CAD build for the part. Positions are in the model's coordinates, mm. Face numbers are marked on the shaded views. A direction names the side the tool comes from. Give positions to 0.01 mm unless a question says otherwise; leave off trailing zeros. Loops run counter-clockwise (first coordinate to the right, second up) from the corner with the lowest first, then second, coordinate; pieces in that order, holes last. Notation, with made-up numbers: (-1, -29) - (26, -29) arc R13 ccw to (26, -6) - close; hole circle Ø3 at (74, 59). An arc over 180 degrees is marked (long way). Return JSON: item names as keys, results as strings.
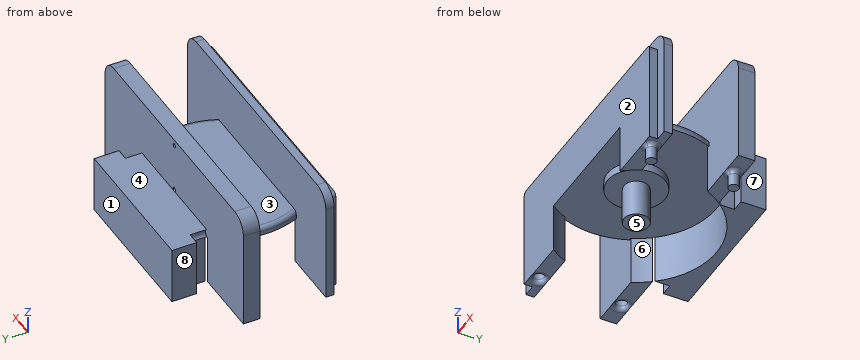
from build123d import *

# Parameters (mm, degrees)
BOSS_EXTRUDE1_DEPTH     = 1
SKETCH2_R               = 1.51
BOSS_EXTRUDE2_DEPTH     = 5.5
SKETCH3_R               = 3.5
BOSS_EXTRUDE3_DEPTH     = 1
SKETCH4_W               = 2
SKETCH4_H               = 17
BOSS_EXTRUDE4_DEPTH     = 6
SKETCH5_W               = 18
SKETCH5_H               = 2
BOSS_EXTRUDE5_DEPTH     = 6
SKETCH6_W               = 7
SKETCH6_H               = 2
BOSS_EXTRUDE6_DEPTH     = 5
BOSS_EXTRUDE7_DEPTH     = 6
CUT_EXTRUDE1_DEPTH      = 21.639767441
SKETCH9_W               = 2.937742252
SKETCH9_H               = 8
CUT_EXTRUDE2_DEPTH      = 6
CUT_EXTRUDE11_START     = -6
SKETCH21_R              = 9.75
SKETCH21_R_2            = 3.5
CUT_EXTRUDE11_DEPTH     = 6
SKETCH10_W              = 32
SKETCH10_H              = 2
BOSS_EXTRUDE8_DEPTH     = 7
FILLET1_R               = 0.5
SKETCH11_R              = 0.625
BOSS_EXTRUDE9_DEPTH     = 2
SKETCH14_W              = 3.5
SKETCH14_H              = 2
CUT_EXTRUDE5_DEPTH      = 24.937418532
SKETCH12_R              = 0.675
CUT_EXTRUDE3_DEPTH      = 2.5
CUT_EXTRUDE6_DEPTH      = 2
FILLET2_R               = 0.5
FILLET3_R               = 0.5
FILLET4_R               = 2
CUT_EXTRUDE7_DEPTH      = 25.677925456
CUT_EXTRUDE7_DEPTH_BACK = 1
SKETCH19_R              = 0.25
CUT_EXTRUDE9_DEPTH      = 2
SKETCH20_W              = 2
SKETCH20_H              = 3
CUT_EXTRUDE10_DEPTH     = 24.937418532


with BuildPart() as part:
    # Sketch1 → Boss-Extrude1 (new body)
    with BuildSketch(Plane.XY):
        Polygon((-11, 6), (-11, 11), (11, 11), (11, 6), (11, -6), (-11, -6), align=None)
    extrude(amount=BOSS_EXTRUDE1_DEPTH)

    # Sketch2 → Boss-Extrude2 (add)
    with BuildSketch(Plane(origin=(0, 0, 0), x_dir=(-1, 0, 0), z_dir=(0, 0, -1))):
        with Locations(Location((0, 0, 0), (0, 0, 180))):
            Circle(SKETCH2_R)
    extrude(amount=BOSS_EXTRUDE2_DEPTH)

    # Sketch3 → Boss-Extrude3 (add)
    with BuildSketch(Plane(origin=(0, 0, 0), x_dir=(-1, 0, 0), z_dir=(0, 0, -1))):
        with Locations(Location((0, 0, 0), (0, 0, 180))):
            Circle(SKETCH3_R)
    extrude(amount=BOSS_EXTRUDE3_DEPTH)

    # Sketch4 → Boss-Extrude4 (add)
    with BuildSketch(Plane(origin=(0, 0, 0), x_dir=(-1, 0, 0), z_dir=(0, 0, -1))):
        with Locations((10, 2.5)):
            Rectangle(SKETCH4_W, SKETCH4_H)
        with Locations((-10, 2.5)):
            Rectangle(SKETCH4_W, SKETCH4_H)
    extrude(amount=BOSS_EXTRUDE4_DEPTH)

    # Sketch5 → Boss-Extrude5 (add)
    with BuildSketch(Plane(origin=(0, 0, 0), x_dir=(-1, 0, 0), z_dir=(0, 0, -1))):
        with Locations((0, 10)):
            Rectangle(SKETCH5_W, SKETCH5_H)
    extrude(amount=BOSS_EXTRUDE5_DEPTH)

    # Sketch6 → Boss-Extrude6 (add)
    with BuildSketch(Plane(origin=(11, 0, 0), x_dir=(0, 0, -1), z_dir=(1, 0, 0))):
        with Locations((2.5, -5)):
            Rectangle(SKETCH6_W, SKETCH6_H)
        with Locations((2.5, 5)):
            Rectangle(SKETCH6_W, SKETCH6_H)
    boss_extrude6 = extrude(amount=BOSS_EXTRUDE6_DEPTH)

    # Mirror1: Boss-Extrude6 across plane
    add(boss_extrude6.mirror(Plane(origin=(0, 0, 0), x_dir=(0, 0, 1), z_dir=(1, 0, 0))))

    # Sketch7 → Boss-Extrude7 (add)
    with BuildSketch(Plane(origin=(0, 0, -6), x_dir=(-1, 0, 0), z_dir=(0, 0, -1))):
        with BuildLine():
            ThreePointArc((-6.708203932, -6), (-8.407551231, -3.211398808), (-9, 0))
            Line((-9, 0), (-9, -6))
            Line((-9, -6), (-6.708203932, -6))
        make_face()
        with BuildLine():
            Line((-9, 9), (-9, 0))
            ThreePointArc((-9, 0), (-6.363961031, 6.363961031), (0, 9))
            Line((0, 9), (-9, 9))
        make_face()
    boss_extrude7 = extrude(amount=-BOSS_EXTRUDE7_DEPTH)

    # Sketch8 → Cut-Extrude1 (cut, through all)
    with BuildSketch(Plane(origin=(0, 0, -6), x_dir=(-1, 0, 0), z_dir=(0, 0, -1))):
        with BuildLine():
            Line((-11, 4), (-9.16515139, 4))
            ThreePointArc((-9.16515139, 4), (-10, 0), (-9.16515139, -4))
            Line((-9.16515139, -4), (-11, -4))
            Line((-11, -4), (-11, 4))
        make_face()
    cut_extrude1 = extrude(amount=-CUT_EXTRUDE1_DEPTH, mode=Mode.SUBTRACT)

    # Sketch9 → Cut-Extrude2 (cut)
    with BuildSketch(Plane(origin=(0, 0, -6), x_dir=(-1, 0, 0), z_dir=(0, 0, -1))):
        with Locations((-9.531128874, 0)):
            Rectangle(SKETCH9_W, SKETCH9_H)
    cut_extrude2 = extrude(amount=-CUT_EXTRUDE2_DEPTH, mode=Mode.SUBTRACT)

    # Mirror2: Boss-Extrude7, Cut-Extrude1, Cut-Extrude2 across plane
    add(boss_extrude7.mirror(Plane(origin=(0, 0, 0), x_dir=(0, 0, 1), z_dir=(1, 0, 0))))
    add(cut_extrude1.mirror(Plane(origin=(0, 0, 0), x_dir=(0, 0, 1), z_dir=(1, 0, 0))), mode=Mode.SUBTRACT)
    add(cut_extrude2.mirror(Plane(origin=(0, 0, 0), x_dir=(0, 0, 1), z_dir=(1, 0, 0))), mode=Mode.SUBTRACT)

    # Sketch21 → Cut-Extrude11 (cut)
    with BuildSketch(Plane(origin=(0, 0, -6), x_dir=(-1, 0, 0), z_dir=(0, 0, -1)).offset(CUT_EXTRUDE11_START)):
        Circle(SKETCH21_R)
        with Locations(Location((0, 0, 0), (0, 0, 180))):
            Circle(SKETCH21_R_2, mode=Mode.SUBTRACT)
    extrude(amount=CUT_EXTRUDE11_DEPTH, mode=Mode.SUBTRACT)

    # Sketch10 → Boss-Extrude8 (add)
    with BuildSketch(Plane.XY.offset(1)):
        with Locations((0, -5)):
            Rectangle(SKETCH10_W, SKETCH10_H)
        with Locations((0, 5)):
            Rectangle(SKETCH10_W, SKETCH10_H)
    extrude(amount=BOSS_EXTRUDE8_DEPTH)

    # Fillet1
    fillet1_edges = [part.edges().sort_by_distance(p)[0] for p in [
        (10, 0, 1),
        (-10, 0, 1),
    ]]
    fillet(fillet1_edges, radius=FILLET1_R)

    # Sketch11 → Boss-Extrude9 (add)
    with BuildSketch(Plane(origin=(0, 0, -6), x_dir=(-1, 0, 0), z_dir=(0, 0, -1))):
        with Locations(Location((-13, -5, 0), (0, 0, 180))):
            Circle(SKETCH11_R)
    boss_extrude9 = extrude(amount=BOSS_EXTRUDE9_DEPTH)

    # Sketch14 → Cut-Extrude5 (cut, through all)
    with BuildSketch(Plane(origin=(0, 0, -6), x_dir=(-1, 0, 0), z_dir=(0, 0, -1))):
        with Locations((9.25, 7)):
            Rectangle(SKETCH14_W, SKETCH14_H)
        with Locations((-9.25, 7)):
            Rectangle(SKETCH14_W, SKETCH14_H)
    extrude(amount=-CUT_EXTRUDE5_DEPTH, mode=Mode.SUBTRACT)

    # Sketch12 → Cut-Extrude3 (cut)
    with BuildSketch(Plane(origin=(0, 0, -6), x_dir=(-1, 0, 0), z_dir=(0, 0, -1))):
        with Locations((13, -5)):
            Circle(SKETCH12_R)
    cut_extrude3 = extrude(amount=-CUT_EXTRUDE3_DEPTH, mode=Mode.SUBTRACT)

    # Sketch16 → Cut-Extrude6 (cut)
    with BuildSketch(Plane(origin=(0, 6, 0), x_dir=(1, 0, 0), z_dir=(0, 1, 0))):
        with BuildLine():
            Line((-7.5, 0), (-7.5, -1))
            ThreePointArc((-7.5, -1), (-7.25, -0.5), (-7.5, 0))
        make_face()
    cut_extrude6 = extrude(amount=CUT_EXTRUDE6_DEPTH, mode=Mode.SUBTRACT)

    # Mirror3: Boss-Extrude9, Cut-Extrude3 across plane
    add(boss_extrude9.mirror(Plane.ZX))
    add(cut_extrude3.mirror(Plane.ZX), mode=Mode.SUBTRACT)

    # Mirror4: Cut-Extrude6 across plane
    add(cut_extrude6.mirror(Plane(origin=(0, 0, 0), x_dir=(0, 0, 1), z_dir=(1, 0, 0))), mode=Mode.SUBTRACT)

    # Fillet2
    fillet2_edges = [part.edges().sort_by_distance(p)[0] for p in [
        (12.375, -5, -6),
        (12.375, 5, -6),
    ]]
    fillet(fillet2_edges, radius=FILLET2_R)

    # Fillet3
    # the kernel refuses this fillet: 0.5 mm, written as the material it takes off along each edge
    with BuildSketch(Plane(origin=(-13, -5, -6), x_dir=(-1, 0, 0), z_dir=(0, -1, 0))) as fillet3_piece_1:
        with BuildLine():
            CenterArc((0.675 + FILLET3_R, -FILLET3_R), FILLET3_R, 90, 90)
            Line((0.675, -FILLET3_R), (0.675, 0))
            Line((0.675, 0), (0.675 + FILLET3_R, 0))
        make_face()
    revolve(axis=Axis((-13, -5, -6), (0, 0, -1)), mode=Mode.SUBTRACT)
    with BuildSketch(Plane(origin=(-13, 5, -6), x_dir=(-1, 0, 0), z_dir=(0, 1, 0))) as fillet3_piece_2:
        with BuildLine():
            CenterArc((0.675 + FILLET3_R, FILLET3_R), FILLET3_R, 180, 90)
            Line((0.675, FILLET3_R), (0.675, 0))
            Line((0.675, 0), (0.675 + FILLET3_R, 0))
        make_face()
    revolve(axis=Axis((-13, 5, -6), (0, 0, 1)), mode=Mode.SUBTRACT)

    # Fillet4
    fillet4_edges = [part.edges().sort_by_distance(p)[0] for p in [
        (16, -5, 8),
        (-16, -5, 8),
        (-16, 5, 8),
        (16, 5, 8),
    ]]
    fillet(fillet4_edges, radius=FILLET4_R)

    # Sketch17 → Cut-Extrude7 (cut, two sides: drawn at the far end of the back side and taken through both)
    with BuildSketch(Plane.XZ.offset(6).offset(-CUT_EXTRUDE7_DEPTH_BACK)):
        with BuildLine():
            Line((-16, 6), (-16, -6))
            Line((-16, -6), (-14.5, -6))
            Line((-14.5, -6), (-14.5, 6))
            ThreePointArc((-14.5, 6), (-14.353553391, 6.353553391), (-14, 6.5))
            Line((-14, 6.5), (14, 6.5))
            ThreePointArc((14, 6.5), (14.353553391, 6.353553391), (14.5, 6))
            Line((14.5, 6), (14.5, -6))
            Line((14.5, -6), (16, -6))
            Line((16, -6), (16, 6))
            ThreePointArc((16, 6), (15.414213562, 7.414213562), (14, 8))
            Line((14, 8), (-14, 8))
            ThreePointArc((-14, 8), (-15.414213562, 7.414213562), (-16, 6))
        make_face()
    extrude(amount=CUT_EXTRUDE7_DEPTH + CUT_EXTRUDE7_DEPTH_BACK, mode=Mode.SUBTRACT)

    # Sketch19 → Cut-Extrude9 (cut)
    with BuildSketch(Plane(origin=(0, 6, 0), x_dir=(1, 0, 0), z_dir=(0, 1, 0))):
        with Locations(Location((0, -1.25, 0), (0, 0, 90))):
            Circle(SKETCH19_R)
        with Locations(Location((0, -7.25, 0), (0, 0, 270))):
            Circle(SKETCH19_R)
    extrude(amount=-CUT_EXTRUDE9_DEPTH, mode=Mode.SUBTRACT)

    # Sketch20 → Cut-Extrude10 (cut, through all)
    with BuildSketch(Plane(origin=(0, 0, -6), x_dir=(-1, 0, 0), z_dir=(0, 0, -1))):
        with Locations((-10, 9.5)):
            Rectangle(SKETCH20_W, SKETCH20_H)
        with Locations((10, 9.5)):
            Rectangle(SKETCH20_W, SKETCH20_H)
    extrude(amount=-CUT_EXTRUDE10_DEPTH, mode=Mode.SUBTRACT)


solid = part.part
1. Cut at C-C, the plane z = -4.25. Give the number of separate pieces and of enclosed holes in the cut face, plus the area to 3 significant figures.
Values follow:
{"separate pieces": "6", "enclosed holes": "2", "area": "106 mm²"}
2. Pull direction Y, two halves, no side cores. Call the marked faces 1, 2, 3 and 4: +Y half, -Y half, draft (parallel to the pull), parting line (faces both ways), or undercut.
Values follow:
{"face 1": "+Y half", "face 2": "-Y half", "face 3": "undercut", "face 4": "draft"}
3. Cut at B-B, the plane x = 11.5. Write the cut outline in (y, z).
Values follow:
{"outline": "(-6, -6) - (-4, -6) - (-4, 8) - (-5, 8) - (-5, 6.5) - (-6, 6.5) - close; (4, -6) - (6, -6) - (6, 8) - (4, 8) - close"}
4. Drill centre lines: probe 1 along Y at (x, z) = (-2.5, 4.5); probe 2 along Y at (x, z) = (-13, -4.45) (3 decimals); probe 3 along Y at (x, z) = (0, -4.5). Where is each one in solid material? Low to high.
Values follow:
{"probe 1": "y = -6 to -4, 4 to 6", "probe 2": "y = -6 to -5.675, -4.325 to -4, 4 to 4.325, 5.675 to 6", "probe 3": "y = -1.51 to 1.51, 9.75 to 11"}
5. Cut at D-D, the plane y = 0. Write the cut outline in (x, z).
Values follow:
{"outline": "(-10, 0) - (-3.5, 0) - (-3.5, -1) - (-1.51, -1) - (-1.51, -5.5) - (1.51, -5.5) - (1.51, -1) - (3.5, -1) - (3.5, 0) - (10, 0) - (10, 0.5) arc R0.5 ccw to (9.5, 1) - (-9.5, 1) arc R0.5 ccw to (-10, 0.5) - close"}
6. Cut at A-A, the plane z = 3. Write the cut outline in (x, y).
Values follow:
{"outline": "(-16, -5) - (-14.5, -5) - (-14.5, -6) - (14.5, -6) - (14.5, -5) - (16, -5) - (16, -4) - (-16, -4) - close; (-16, 4) - (16, 4) - (16, 6) - (-16, 6) - close"}
7. Drop flat-ended pins along their axis: P1, Ø1.9, axis at y = 7, z = -1.5, coming from the -X side; P2, Ø8, axis at x = 8.5, y = 2, coming from the -Z side; P3, Ø5, axis at x = 1, y = -0.5, coming from the -Z side. Give the stop position or say it passes through.
Values follow:
{"P1": "stops at x = -7.5", "P2": "stops at z = -6", "P3": "stops at z = -5.5"}
8. Which spindle directions (+Z, -Z, +X, -X, +Y, -Y) get a long thin tool onto all of the face, cutting with end or side? Do the marked faces 5, 6, 7 and 8. Say none if no direction does.
Values follow:
{"face 5": "-Z, +X, -X, -Y", "face 6": "-Z", "face 7": "+Z, -Z, +X, +Y", "face 8": "+Z, -Z, -X, +Y"}
